```python
from build123d import *

# Parameters (mm, degrees)
F0_R     = 10.16
F1_DEPTH = 15.24
F2_R     = 2.54
F3_R     = 1.397
F4_DEPTH = 10.16


with BuildPart() as f1:
    # F0 (on Top) → F1 (new body)
    with BuildSketch(Plane.XY):
        Circle(F0_R)
    extrude(amount=F1_DEPTH)

    # F2
    f2_edges = [f1.edges().sort_by_distance(p)[0] for p in [
        (-10.16, 0, 0),
        (-10.16, 0, 15.24),
    ]]
    fillet(f2_edges, radius=F2_R)

    # F3 (on face) → F4 (cut)
    with BuildSketch(Plane.XY.offset(15.24)):
        Circle(F3_R)
    extrude(amount=-F4_DEPTH, mode=Mode.SUBTRACT)


solid = f1.part
```
Check sheet for the modelled part. Datum: model origin and axes. Units: mm. A direction names the side the tool comes from. Round coordinates to 2 decimals unless told otherwise and drop trailing zeros. Loops run counter-clockwise (first coordinate to the right, second up) from the corner with the lowest first, then second, coordinate; pieces in that order, holes last. Notation, with made-up numbers: (88, -3) - (103, -3) arc R10 ccw to (103, 12) - close; hole circle Ø4 at (63, -28.75). An arc over 180 degrees is marked (long way). Write item = value, one per line. Start each with the question number.
Q1. Release check for a two-part mould opening along X. For faces 3 (the face through (0, 0, 0)), 4 (the face through (-1.323, 10.074, 7.549)), 5 (the face through (-1.11, -0.85, 10.23)) record: pulls with the +X half, pulls with the -X half, needs draft (parallel to the pull), parting line crosses it, or undercut.
Q2. Section check C-C (z = 9.5). Record the boundary of the cut face in (x, y), plus the area to 3 significant figures.
Q3. Depth check by flat-ended pin: P1, Ø2.5, axis at x = 0, y = 0, coming from the +Z side; P2, Ø6, axis at x = -7, z = 13.5, coming from the -Y side; P3, Ø2, axis at y = -6, z = 12, coming from the -X side. Enter the tip coordinate at first touch or a pass-through.
Q4. Section check D-D (z = 4.25). Record the boundary of the cut face in (x, y).
Q5. Thickness scan on L1, parallel to Y at x = 0, z = 7.75; L2, parallel to X at y = -3, z = 12; L3, parallel to Y at x = 6.25, z = 14. Record the ranges inside material, lowest first.
Q6. Section check A-A (y = 0). Record the boundary of the cut face in (x, z).
Q7. Access from +Z, -Z, +X, -X, +Y, -Y to the whole of each face (thin tool, end or side, straight path). Record for faces 1 (the face through (2, 0, 15.24)), 2 (the face through (0, 0, 5.08)).
Derived:
q1.face_3 = needs draft
q1.face_4 = parting line crosses it
q1.face_5 = undercut
q2.outline = circle Ø20.32 at (0, 0); hole circle Ø2.79 at (0, 0)
q2.area = 318 mm^2
q3.P1 = 5.08
q3.P2 = -9.3
q3.P3 = -8.84
q4.outline = circle Ø20.32 at (0, 0)
q5.L1 = -10.16 to -1.4, 1.4 to 10.16
q5.L2 = -9.71 to 9.71
q5.L3 = -7.55 to 7.55
q6.outline = (-10.16, 2.54) arc R2.54 ccw to (-7.62, 0) - (7.62, 0) arc R2.54 ccw to (10.16, 2.54) - (10.16, 12.7) arc R2.54 ccw to (7.62, 15.24) - (1.4, 15.24) - (1.4, 5.08) - (-1.4, 5.08) - (-1.4, 15.24) - (-7.62, 15.24) arc R2.54 ccw to (-10.16, 12.7) - close
q7.face_1 = +Z, +X, -X, +Y, -Y
q7.face_2 = +Z
